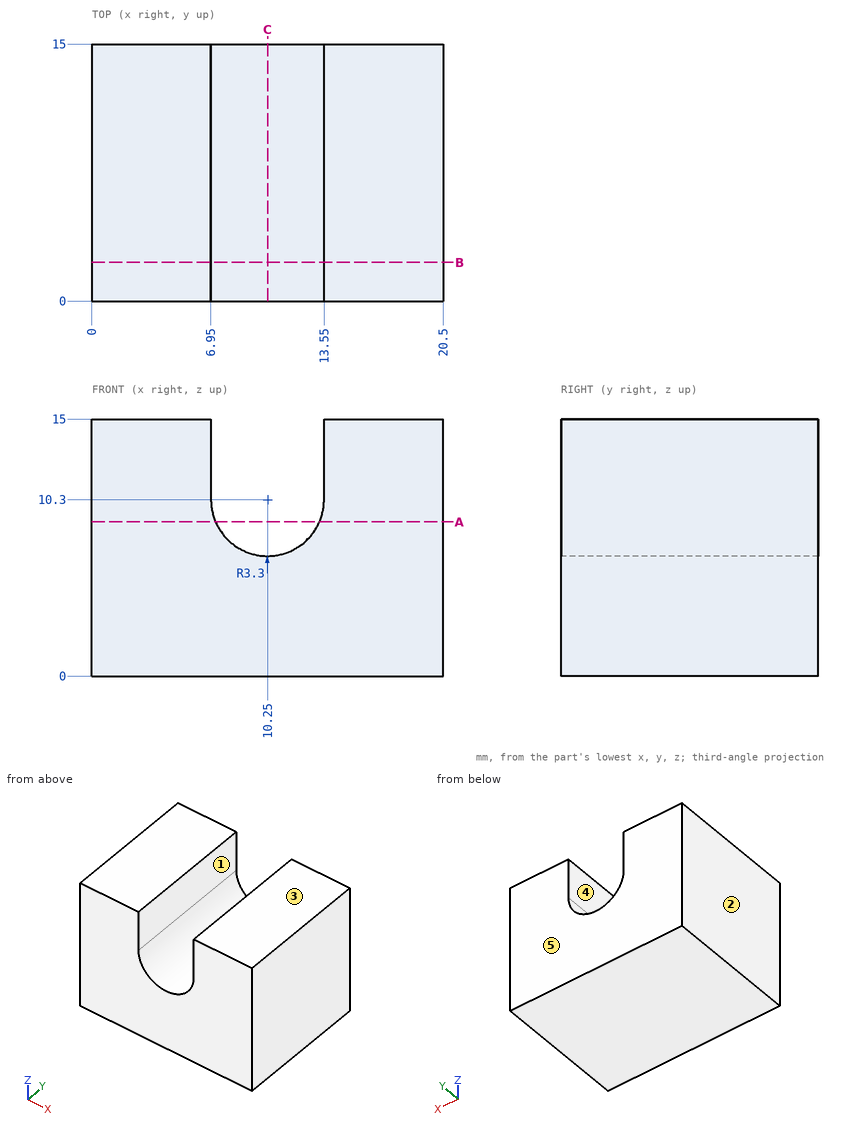
The drawing under review shows one solid part. Ordinate dimensions are in mm from its lowest x, y, z. A direction names the side the tool comes from. Round coordinates to 2 decimals unless told otherwise and drop trailing zeros. Loops run counter-clockwise (first coordinate to the right, second up) from the corner with the lowest first, then second, coordinate; pieces in that order, holes last. Notation, with made-up numbers: M 81,63.25 L 91,63.25 A31 cw 91,90.25 Z; hole C -5.5,13.5 d1. An arc over 180 degrees is marked long. Answer as CSV lines item,"result". Start each with the question number.
Item 1: Insertion check: P1, Ø5, axis at y = 8, z = 11.5, coming from the -X side; P2, Ø1.5, axis at x = 9, y = 4.5, coming from the +Z side. Each pin has a flat end and moves straight along its axis. Give the tip position at first contact, or say it passes through.
Item 2: For the marked faces 4 and 5, list the 3-axis set-ups (+Z, -Z, +X, -X, +Y, -Y) from which the entire face can be reached by the end or side of a thin tool; tool diameter is ignored.
Item 3: Wall thickness on line 1 (X direction, y = 7.25, z = 12); line 2 (X direction, y = 1.25, z = 10); line 3 (Z direction, x = 10.25, y = 5.5): over which ranges is each line inside the solid? List them lowest first. Write a range as [from, to].
Item 4: Mouldability with a two-part tool opening along X and no side actions: class the marked faces 1, 2 and 3 as released by +X, released by -X, zero draft, split by the parting line, or undercut.
Item 5: Consider section B-B (y = 2.25). Write out the cut boundary in (x, z), then the cut area to 3 significant figures.
Item 6: Consider section A-A (z = 9). Write out the cut boundary in (x, y).
Item 7: Consider section C-C (x = 10.25). Write out the cut boundary in (y, z).
Answer:
1,P1,"stops at x = 0"
1,P2,"stops at z = 7.68"
2,face 4,"+Z, +Y, -Y"
2,face 5,"+Z, -Z, +X, -X, +Y"
3,line 1,"x = [0, 6.95], [13.55, 20.5]"
3,line 2,"x = [0, 6.96], [13.54, 20.5]"
3,line 3,"z = [0, 7]"
4,face 1,"undercut"
4,face 2,"released by -X"
4,face 3,"zero draft"
5,outline,"M 0,0 L 20.5,0 L 20.5,15 L 13.55,15 L 13.55,10.3 A3.3 cw 6.95,10.3 L 6.95,15 L 0,15 Z"
5,area,"259 mm^2"
6,outline,"M 0,0 L 7.22,0 L 7.22,15 L 0,15 Z; M 13.28,0 L 20.5,0 L 20.5,15 L 13.28,15 Z"
7,outline,"M 0,0 L 15,0 L 15,7 L 0,7 Z"
